CAD build for the part. Positions are in the model's coordinates, mm. Coordinates: 2 decimals unless noted, no trailing zeros. Write each question's results on one line, items separated by ' | '.
Autodesk Inventor part; units mm, degrees
ref_plane "C1_XY" through (0, 0, 0) normal (0, 0, 1) x (1, 0, 0)
ref_plane "C1_YZ" through (0, 0, 0) normal (1, 0, 0) x (0, 1, 0)
ref_plane "C1_ZX" through (0, 0, 0) normal (0, 1, 0) x (0, 0, 1)
sketch "Sketch_60" plane through (0, 0, 0) normal (0, 0, 1) x (1, 0, 0)
  arc A0 (-30, -27) -> (-27, -30) centre (-27, -27) ccw
  line L0 (-27, -30) -> (-5, -30)
  line L1 (-5, -30) -> (-5, -24)
  line L2 (-5, -24) -> (-10, -24)
  line L3 (-10, -24) -> (-10, -19.6167)
  line L4 (-10, -19.6167) -> (-7.3833, -17)
  line L5 (-7.3833, -17) -> (-3.3464, -17)
  line L6 (-3.3464, -17) -> (-3, -16.8)
  line L7 (-3, -16.8) -> (-2.6536, -17)
  line L8 (-2.6536, -17) -> (-1.2124, -17)
  line L9 (-1.2124, -17) -> (0, -16.3)
  line L10 (0, -16.3) -> (1.2124, -17)
  line L11 (1.2124, -17) -> (2.6536, -17)
  line L12 (2.6536, -17) -> (3, -16.8)
  line L13 (3, -16.8) -> (3.3464, -17)
  line L14 (3.3464, -17) -> (7.3833, -17)
  line L15 (7.3833, -17) -> (10, -19.6167)
  line L16 (10, -19.6167) -> (10, -24)
  line L17 (10, -24) -> (5, -24)
  line L18 (5, -24) -> (5, -30)
  line L19 (5, -30) -> (27, -30)
  arc A1 (27, -30) -> (30, -27) centre (27, -27) ccw
  line L20 (30, -27) -> (30, -5)
  line L21 (30, -5) -> (24, -5)
  line L22 (24, -5) -> (24, -10)
  line L23 (24, -10) -> (19.6167, -10)
  line L24 (19.6167, -10) -> (17, -7.3833)
  line L25 (17, -7.3833) -> (17, -3.3464)
  line L26 (17, -3.3464) -> (16.8, -3)
  line L27 (16.8, -3) -> (17, -2.6536)
  line L28 (17, -2.6536) -> (17, -1.2124)
  line L29 (17, -1.2124) -> (16.3, 0)
  line L30 (16.3, 0) -> (17, 1.2124)
  line L31 (17, 1.2124) -> (17, 2.6536)
  line L32 (17, 2.6536) -> (16.8, 3)
  line L33 (16.8, 3) -> (17, 3.3464)
  line L34 (17, 3.3464) -> (17, 7.3833)
  line L35 (17, 7.3833) -> (19.6167, 10)
  line L36 (19.6167, 10) -> (24, 10)
  line L37 (24, 10) -> (24, 5)
  line L38 (24, 5) -> (30, 5)
  line L39 (30, 5) -> (30, 27)
  arc A2 (30, 27) -> (27, 30) centre (27, 27) ccw
  line L40 (27, 30) -> (5, 30)
  line L41 (5, 30) -> (5, 24)
  line L42 (5, 24) -> (10, 24)
  line L43 (10, 24) -> (10, 19.6167)
  line L44 (10, 19.6167) -> (7.3833, 17)
  line L45 (7.3833, 17) -> (3.3464, 17)
  line L46 (3.3464, 17) -> (3, 16.8)
  line L47 (3, 16.8) -> (2.6536, 17)
  line L48 (2.6536, 17) -> (1.2124, 17)
  line L49 (1.2124, 17) -> (0, 16.3)
  line L50 (0, 16.3) -> (-1.2124, 17)
  line L51 (-1.2124, 17) -> (-2.6536, 17)
  line L52 (-2.6536, 17) -> (-3, 16.8)
  line L53 (-3, 16.8) -> (-3.3464, 17)
  line L54 (-3.3464, 17) -> (-7.3833, 17)
  line L55 (-7.3833, 17) -> (-10, 19.6167)
  line L56 (-10, 19.6167) -> (-10, 24)
  line L57 (-10, 24) -> (-5, 24)
  line L58 (-5, 24) -> (-5, 30)
  line L59 (-5, 30) -> (-27, 30)
  arc A3 (-27, 30) -> (-30, 27) centre (-27, 27) ccw
  line L60 (-30, 27) -> (-30, 5)
  line L61 (-30, 5) -> (-24, 5)
  line L62 (-24, 5) -> (-24, 10)
  line L63 (-24, 10) -> (-19.6167, 10)
  line L64 (-19.6167, 10) -> (-17, 7.3833)
  line L65 (-17, 7.3833) -> (-17, 3.3464)
  line L66 (-17, 3.3464) -> (-16.8, 3)
  line L67 (-16.8, 3) -> (-17, 2.6536)
  line L68 (-17, 2.6536) -> (-17, 1.2124)
  line L69 (-17, 1.2124) -> (-16.3, 0)
  line L70 (-16.3, 0) -> (-17, -1.2124)
  line L71 (-17, -1.2124) -> (-17, -2.6536)
  line L72 (-17, -2.6536) -> (-16.8, -3)
  line L73 (-16.8, -3) -> (-17, -3.3464)
  line L74 (-17, -3.3464) -> (-17, -7.3833)
  line L75 (-17, -7.3833) -> (-19.6167, -10)
  line L76 (-19.6167, -10) -> (-24, -10)
  line L77 (-24, -10) -> (-24, -5)
  line L78 (-24, -5) -> (-30, -5)
  line L79 (-30, -5) -> (-30, -27)
  circle A4 centre (20, 20) radius 3.5
  circle A5 centre (20, -20) radius 3.5
  circle A6 centre (-20, 20) radius 3.5
  circle A7 centre (-20, -20) radius 3.5
extrude "Extrusion1" add sketch "Sketch_60" against normal blind 1066.8
sketch "Sketch2" plane through (0, 0, -1066.8) normal (0, 0, -1) x (-1, 0, 0)
  point P0 (0, 0)
hole "Hole1" at (0, 0, -1066.8) direction (0, 0, 1) diameter 10.5 depth 1000
ref_plane "C1_XY" through (0, 0, 0) normal (0, 0, 1) x (1, 0, 0)
ref_plane "C1_YZ" through (0, 0, 0) normal (1, 0, 0) x (0, 1, 0)
ref_plane "C1_ZX" through (0, 0, 0) normal (0, 1, 0) x (0, 0, 1)
ref_plane "to_frame_cap1_XY" through (0, 0, 0) normal (0, 0, 1) x (1, 0, 0)
ref_plane "to_frame_cap1_YZ" through (0, 0, 0) normal (1, 0, 0) x (0, 1, 0)
ref_plane "to_frame_cap1_ZX" through (0, 0, 0) normal (0, 1, 0) x (0, 0, 1)
ref_plane "to_frame_cap2_XY" through (0, 0, -1000) normal (0, 0, -1) x (1, 0, 0)
ref_plane "to_frame_cap2_YZ" through (0, 0, -1000) normal (1, 0, 0) x (0, -1, 0)
ref_plane "to_frame_cap2_ZX" through (0, 0, -1000) normal (0, -1, 0) x (0, 0, -1)
properties part number "6060-3.5"
1) Slice it at A-A (z = -865). Count the separate pieces of the cut face and the enclosed holes in it, then the cut area to 3 significant figures.
Outcome:
separate pieces: 1 | enclosed holes: 5 | area: 2,580 mm^2
2) Drill centre lines: L1, parallel to Y at x = 20, z = -788; L2, parallel to X at y = -21, z = -356; L3, parallel to Y at x = 0, z = -371.5. Where is each one in solid material? Low to high. Write a range as from..to.
Outcome:
L1: y = -30..-23.5, -16.5..-10, 10..16.5, 23.5..30 | L2: x = -30..-23.35, -16.65..-10, 10..16.65, 23.35..30 | L3: y = -16.3..-5.25, 5.25..16.3
3) Two-plate mould, pull along Y, no slides. Class faces 1 (the flat face through (30, 16, -526)), 2 (the flat face through (16, -30, -526)), 3 (the flat face through (-16, 30, -526)): pulls with the +Y half, pulls with the -Y half, needs draft (parallel to the pull), parting line crosses it, or undercut.
Outcome:
face 1: needs draft | face 2: pulls with the -Y half | face 3: pulls with the +Y half
4) Pin check, flat tips, straight feed: pin 1 (0.7 mm diameter, centred on x = 1.5, z = -546.5, fed in from -Y); pin 2 (5 mm diameter, centred on x = 0.5, z = -738.5, fed in from +Y). Stop position of each tip, or through.
Outcome:
pin 1: stops at y = -17 | pin 2: stops at y = 17
